The drawing under review shows one solid part. Ordinate dimensions are in mm from its lowest x, y, z. A direction names the side the tool comes from. Give positions to 0.01 mm unless a question says otherwise; leave off trailing zeros. Loops run counter-clockwise (first coordinate to the right, second up) from the corner with the lowest first, then second, coordinate; pieces in that order, holes last.
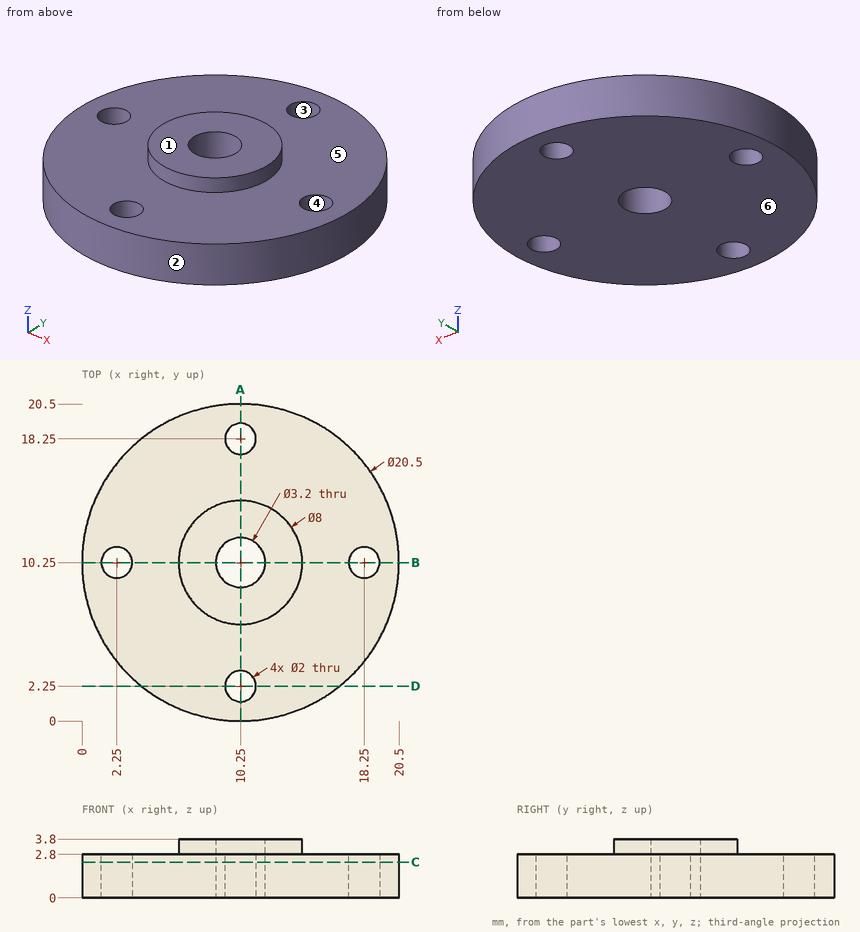
Item 1: Tool access review of the marked faces 5 and 6: name each direction out of +Z, -Z, +X, -X, +Y, -Y from which nothing blocks a thin tool from reaching the whole face with its end or side.
Answer:
face 5: +Z
face 6: -Z, +X, -X, +Y, -Y
Item 2: Take a section at C-C on z = 2.3. Give the boundary of the cut face in (x, y).
Answer:
outline: circle Ø20.5 at (10.25, 10.25); hole circle Ø2 at (2.25, 10.25); hole circle Ø3.2 at (10.25, 10.25); hole circle Ø2 at (10.25, 2.25); hole circle Ø2 at (10.25, 18.25); hole circle Ø2 at (18.25, 10.25)
Item 3: Clearance check with flat-ended pins moving along their axes: pin 1 Ø2.5 at (x, y) = (10.25, 2.25) entering from +Z; pin 2 Ø1 at (x, z) = (11, 1) entering from -Y; pin 3 Ø1.8 at (x, y) = (10.25, 18.25) entering from -Z. State where each tip first meets the part, or that it passes through.
Answer:
pin 1: stops at z = 2.8
pin 2: stops at y = 0
pin 3: passes through
Item 4: For L1, parallel to Y at x = 10.25, z = 1.35; L2, parallel to Z at x = 17.25, y = 11; L3, parallel to Y at x = 18, z = 2.6, list the stretches that pass through material, from the lowest coordinate up.
Answer:
L1: y = 0 to 1.25, 3.25 to 8.65, 11.85 to 17.25, 19.25 to 20.5
L2: z = 0 to 2.8
L3: y = 3.54 to 9.28, 11.22 to 16.96
Item 5: Take a section at D-D on y = 2.25. Give the boundary of the cut face in (x, z), and give its area (3 significant figures).
Answer:
outline: (3.84, 0) - (9.25, 0) - (9.25, 2.8) - (3.84, 2.8) - close; (11.25, 0) - (16.66, 0) - (16.66, 2.8) - (11.25, 2.8) - close
area: 30.3 mm2
Item 6: Take a section at A-A on x = 10.25. Give the boundary of the cut face in (y, z), and give its area (3 significant figures).
Answer:
outline: (0, 0) - (1.25, 0) - (1.25, 2.8) - (0, 2.8) - close; (3.25, 0) - (8.65, 0) - (8.65, 3.8) - (6.25, 3.8) - (6.25, 2.8) - (3.25, 2.8) - close; (11.85, 0) - (17.25, 0) - (17.25, 2.8) - (14.25, 2.8) - (14.25, 3.8) - (11.85, 3.8) - close; (19.25, 0) - (20.5, 0) - (20.5, 2.8) - (19.25, 2.8) - close
area: 42.0 mm2
Item 7: The part is to be moulded in two halves that separate along Y. For the marked faces 1, 2, 3 and 4, say which applies: released by +Y, released by -Y, zero draft, split by the parting line, or undercut.
Answer:
face 1: zero draft
face 2: split by the parting line
face 3: undercut
face 4: undercut
